from build123d import *

# Parameters (mm, degrees)
CYLINDER008_R         = 1.9
CYLINDER008_DEPTH     = 10
CYLINDER007_R         = 1.9
CYLINDER007_DEPTH     = 10
CYLINDER009_R         = 1.9
CYLINDER009_DEPTH     = 10
CYLINDER006_R         = 1.9
CYLINDER006_DEPTH     = 10
CYLINDER010_R         = 1.65
CYLINDER010_DEPTH     = 10
BOX025_W              = 13
BOX025_H              = 14
BOX025_DEPTH          = 31
CYLINDER004_R         = 5
CYLINDER004_DEPTH     = 40
BOX023_W              = 46
BOX023_H              = 4
BOX023_DEPTH          = 40
BOX024_W              = 56
BOX024_H              = 7
BOX024_DEPTH          = 40
CHAMFER006006007_SIZE = 4
CHAMFER006006008_SIZE = 3
CHAMFER006006009_SIZE = 1
CHAMFER006006010_SIZE = 0.4


with BuildPart() as cylinder008:
    # Cylinder008 → Cylinder008 (new body)
    with BuildSketch(Plane(origin=(37.5, -9, 33), x_dir=(1, 0, 0), z_dir=(0, 1, 0))):
        Circle(CYLINDER008_R)
    extrude(amount=CYLINDER008_DEPTH)


with BuildPart() as cylinder007:
    # Cylinder007 → Cylinder007 (new body)
    with BuildSketch(Plane(origin=(15, -9, 20), x_dir=(1, 0, 0), z_dir=(0, 1, 0))):
        Circle(CYLINDER007_R)
    extrude(amount=CYLINDER007_DEPTH)


with BuildPart() as fusion002:
    # Cylinder009 → Cylinder009 (new body)
    with BuildSketch(Plane(origin=(37.5, -9, 7), x_dir=(1, 0, 0), z_dir=(0, 1, 0))):
        Circle(CYLINDER009_R)
    extrude(amount=CYLINDER009_DEPTH)

    # Fusion002: union Cylinder008, Cylinder007
    add(cylinder008.part)
    add(cylinder007.part)


with BuildPart() as cylinder006:
    # Cylinder006 → Cylinder006 (new body)
    with BuildSketch(Plane(origin=(-6, -1, 0), x_dir=(1, 0, 0), z_dir=(0, 0, 1))):
        Circle(CYLINDER006_R)
    extrude(amount=CYLINDER006_DEPTH)


with BuildPart() as fusion004:
    # Cylinder010 → Cylinder010 (new body)
    with BuildSketch(Plane(origin=(-6, -1, 30), x_dir=(1, 0, 0), z_dir=(0, 0, 1))):
        Circle(CYLINDER010_R)
    extrude(amount=CYLINDER010_DEPTH)

    # Fusion003: union Cylinder006
    add(cylinder006.part)

    # Fusion004: union Fusion002
    add(fusion002.part)


with BuildPart() as cube024:
    # Box025 → Box025 (new body)
    with BuildSketch(Plane(origin=(-12, -9, 4.5), x_dir=(1, 0, 0), z_dir=(0, 0, 1))):
        with Locations((6.5, 7)):
            Rectangle(BOX025_W, BOX025_H)
    extrude(amount=BOX025_DEPTH)


with BuildPart() as cylinder004:
    # Cylinder004 → Cylinder004 (new body)
    with BuildSketch(Plane(origin=(-6, -1, 0), x_dir=(1, 0, 0), z_dir=(0, 0, 1))):
        Circle(CYLINDER004_R)
    extrude(amount=CYLINDER004_DEPTH)


with BuildPart() as cube022:
    # Box023 → Box023 (new body)
    with BuildSketch(Plane(origin=(4.5, -4, 0), x_dir=(1, 0, 0), z_dir=(0, 0, 1))):
        with Locations((23, 2)):
            Rectangle(BOX023_W, BOX023_H)
    extrude(amount=BOX023_DEPTH)


with BuildPart() as chamfer006006010:
    # Box024 → Box024 (new body)
    with BuildSketch(Plane(origin=(-11, -8, 0), x_dir=(1, 0, 0), z_dir=(0, 0, 1))):
        with Locations((28, 3.5)):
            Rectangle(BOX024_W, BOX024_H)
    extrude(amount=BOX024_DEPTH)

    # Chamfer006006007
    chamfer006006007_edges = [chamfer006006010.edges().sort_by_distance(p)[0] for p in [
        (-11, -8, 20),
    ]]
    chamfer(chamfer006006007_edges, length=CHAMFER006006007_SIZE)

    # Cut002002: cut Cube022
    add(cube022.part, mode=Mode.SUBTRACT)

    # Chamfer006006008
    chamfer006006008_edges = [chamfer006006010.edges().sort_by_distance(p)[0] for p in [
        (45, -6, 40),
        (45, -6, 0),
    ]]
    chamfer(chamfer006006008_edges, length=CHAMFER006006008_SIZE)

    # Fusion001: union Cylinder004
    add(cylinder004.part)

    # Cut002003: cut Cube024
    add(cube024.part, mode=Mode.SUBTRACT)

    # Chamfer006006009
    chamfer006006009_edges = [chamfer006006010.edges().sort_by_distance(p)[0] for p in [
        (1, -8, 20),
    ]]
    chamfer(chamfer006006009_edges, length=CHAMFER006006009_SIZE)

    # Cut002004: cut Fusion004
    add(fusion004.part, mode=Mode.SUBTRACT)

    # Chamfer006006010
    chamfer006006010_edges = [chamfer006006010.edges().sort_by_distance(p)[0] for p in [
        (17.5, -8, 40),
        (43.5, -8, 38.5),
        (45, -8, 20),
        (17.5, -8, 0),
        (43.5, -8, 1.5),
        (13.1, -8, 20),
        (35.6, -8, 7),
        (35.6, -8, 33),
        (-9, -6, 40),
        (43.5, -4, 38.5),
        (-9, -6, 0),
        (45, -4, 20),
        (43.5, -4, 1.5),
        (1.75, -1, 0),
        (1.75, -1, 40),
        (-6, 4, 40),
        (-11, -2.5, 40),
        (-6, 0.65, 40),
        (-6, -2.65, 40),
        (-6, 4, 0),
        (-11, -2.5, 0),
        (-6, -2.9, 0),
        (-6, 0.9, 0),
        (4.5, -2.5, 40),
        (4.5, -2.5, 0),
        (23.25, -4, 0),
        (23.25, -4, 40),
    ]]
    chamfer(chamfer006006010_edges, length=CHAMFER006006010_SIZE)


solid = chamfer006006010.part
Source: CAD feature listing. Evaluate the final solid. Frame: model axes, mm. A direction names the side the tool comes from. Coordinates: 2 decimals unless noted, no trailing zeros. Order: outer loops, then holes, each group sorted by start corner. A loop starts at its lowest first (then second) coordinate and runs counter-clockwise, first axis right, second up.
Item 1: Cut plane D-D (x = -6). Return loops of the section in (y, z), plus the area to 3 significant figures.
Output values:
outline: (-8, 0.4) - (-7.6, 0) - (-3.3, 0) - (-2.9, 0.4) - (-2.9, 4.5) - (-8, 4.5) - close; (-8, 35.5) - (-2.65, 35.5) - (-2.65, 39.6) - (-3.05, 40) - (-7.6, 40) - (-8, 39.6) - close; (0.65, 35.5) - (4, 35.5) - (4, 39.6) - (3.6, 40) - (1.05, 40) - (0.65, 39.6) - close; (0.9, 0.4) - (1.3, 0) - (3.6, 0) - (4, 0.4) - (4, 4.5) - (0.9, 4.5) - close
area: 75.4 mm2
Item 2: Cut plane B-B (x = 15). Return loops of the section in (y, z), plus the area to 3 significant figures.
Output values:
outline: (-8, 0.4) - (-7.6, 0) - (-4.4, 0) - (-4, 0.4) - (-4, 18.1) - (-7.6, 18.1) - (-8, 17.7) - close; (-8, 22.3) - (-7.6, 21.9) - (-4, 21.9) - (-4, 39.6) - (-4.4, 40) - (-7.6, 40) - (-8, 39.6) - close
area: 144 mm2
Item 3: Cut plane A-A (z = 20). Return loops of the section in (x, y), plus the area to 3 significant figures.
Output values:
outline: (1, -7) - (2, -8) - (12.7, -8) - (13.1, -7.6) - (13.1, -4) - (4.5, -4) - (4.5, -1) - (1, -1) - close; (16.9, -7.6) - (17.3, -8) - (44.6, -8) - (45, -7.6) - (45, -4.4) - (44.6, -4) - (16.9, -4) - close
area: 170 mm2
Item 4: Pull-direction query (Y, two-part tool) for faces 3 (the face through (43.34, -7.8, 38.38)), 4 (the face through (-7.65, -0.93, 37.52)), 5 (the face through (39.255, -5.825, 33.728)), 6 (the face through (43.34, -4.2, 38.38)); classes: pulls with the +Y half, pulls with the -Y half, needs draft (parallel to the pull), parting line crosses it, or undercut.
Output values:
face 3: pulls with the -Y half
face 4: undercut
face 5: needs draft
face 6: pulls with the +Y half
Item 5: Set-up query: faces 1 (the face through (24, -4, 20)), 2 (the face through (-9, -6, 38)). Return all of +Z, -Z, +X, -X, +Y, -Y with unobstructed straight access to the full face (end or side cutting, diameter ignored); none if empty.
Output values:
face 1: +Z, -Z, +X, +Y
face 2: +Z, -Z, -X, -Y
Item 6: Cut plane C-C (x = 37.5). Return loops of the section in (y, z).
Output values:
outline: (-8, 0.4) - (-7.6, 0) - (-4.4, 0) - (-4, 0.4) - (-4, 5.1) - (-7.6, 5.1) - (-8, 4.7) - close; (-8, 9.3) - (-7.6, 8.9) - (-4, 8.9) - (-4, 31.1) - (-7.6, 31.1) - (-8, 30.7) - close; (-8, 35.3) - (-7.6, 34.9) - (-4, 34.9) - (-4, 39.6) - (-4.4, 40) - (-7.6, 40) - (-8, 39.6) - close
Item 7: Material intervals for line 1 (Z direction, x = 37.5, y = -4.7); line 2 (Z direction, x = 15, y = -6.25); line 3 (Y direction, x = -6, z = 2.1), sorted ascending.
Output values:
line 1: z = 0 to 5.1, 8.9 to 31.1, 34.9 to 40
line 2: z = 0 to 18.1, 21.9 to 40
line 3: y = -8 to -2.9, 0.9 to 4
Item 8: First-contact query: P1, Ø12, axis at x = 27, z = 13, coming from the +Y side; P2, Ø4, axis at x = -6, y = -1, coming from the +Z side; P3, Ø3.5, axis at x = 37.5, z = 33, coming from the -Y side; P4, Ø1.5, axis at y = -1, z = 31.5, coming from the -X side. Flat tips, straight axial feed; report the tip coordinate or a pass-through.
Output values:
P1: stops at y = -4
P2: stops at z = 39.95
P3: passes through
P4: stops at x = 1
